CAD build for the part. Positions are in the model's coordinates, mm. A direction names the side the tool comes from. Coordinates: 2 decimals unless noted, no trailing zeros. Loops run counter-clockwise (first coordinate to the right, second up) from the corner with the lowest first, then second, coordinate; pieces in that order, holes last. Notation, with made-up numbers: (-37, -20.75) -> (-23, -20.75) arc R30 cw to (-23, 5.25) -> close; hole circle Ø9 at (52.25, 3.5). An arc over 180 degrees is marked (long way). Answer as a JSON object with one key per item and string values. Group by question number.
from build123d import *

# Parameters (mm, degrees)
SKETCH1_W           = 105.7
SKETCH1_H           = 105.7
SKETCH1_R           = 22.5
BOSS_EXTRUDE1_DEPTH = 10
SKETCH3_W           = 102
SKETCH3_H           = 102
SKETCH3_W_2         = 93
SKETCH3_H_2         = 93
CUT_EXTRUDE1_DEPTH  = 5
SKETCH8_R           = 3
CUT_EXTRUDE5_DEPTH  = 76.407194617
SKETCH4_R           = 10.375
CUT_EXTRUDE7_DEPTH  = 76.407194617
CUT_EXTRUDE11_DEPTH = 76.407194617
BOSS_EXTRUDE5_START = -40
SKETCH9_R           = 3
BOSS_EXTRUDE5_DEPTH = 40
CUT_EXTRUDE12_DEPTH = 47
CUT_EXTRUDE13_DEPTH = 2.5


with BuildPart() as part:
    # Sketch1 → Boss-Extrude1 (new body)
    with BuildSketch(Plane(origin=(0, 0, 0), x_dir=(1, 0, 0), z_dir=(0, 1, 0))):
        Rectangle(SKETCH1_W, SKETCH1_H)
        with Locations(Location((0, 0, 0), (0, 0, 270))):
            Circle(SKETCH1_R, mode=Mode.SUBTRACT)
    extrude(amount=BOSS_EXTRUDE1_DEPTH)

    # Sketch3 → Cut-Extrude1 (cut)
    with BuildSketch(Plane(origin=(0, 10, 0), x_dir=(1, 0, 0), z_dir=(0, 1, 0))):
        Rectangle(SKETCH3_W, SKETCH3_H)
        Rectangle(SKETCH3_W_2, SKETCH3_H_2, mode=Mode.SUBTRACT)
    extrude(amount=-CUT_EXTRUDE1_DEPTH, mode=Mode.SUBTRACT)

    # Sketch8 → Cut-Extrude5 (cut, through all)
    with BuildSketch(Plane.XZ.offset(-10)):
        with Locations(Location((-31.819805153, 31.819805153, 0), (0, 0, 270))):
            Circle(SKETCH8_R)
    extrude(amount=CUT_EXTRUDE5_DEPTH, mode=Mode.SUBTRACT)

    # Sketch4 → Cut-Extrude7 (cut, through all)
    with BuildSketch(Plane(origin=(0, 10, 0), x_dir=(1, 0, 0), z_dir=(0, 1, 0))):
        with Locations(Location((28.284271247, 28.284271247, 0), (0, 0, 270))):
            Circle(SKETCH4_R)
    extrude(amount=-CUT_EXTRUDE7_DEPTH, mode=Mode.SUBTRACT)

    # Sketch12 → Cut-Extrude11 (cut, through all)
    with BuildSketch(Plane.XZ):
        Polygon((43.899242251, -32.468290118), (39.71522338, -16.853319114), (24.100252377, -12.669300244), (12.669300244, -24.100252377), (16.853319114, -39.71522338), (32.468290118, -43.899242251), align=None)
    extrude(amount=-CUT_EXTRUDE11_DEPTH, mode=Mode.SUBTRACT)

    # Sketch9 → Boss-Extrude5 (add)
    with BuildSketch(Plane.XZ.offset(-10).offset(BOSS_EXTRUDE5_START)):
        Polygon((-23.44822625, 31.819805153), (-27.634015702, 39.069805153), (-36.005594605, 39.069805153), (-40.191384057, 31.819805153), (-36.005594605, 24.569805153), (-27.634015702, 24.569805153), align=None)
        with Locations(Location((-31.819805153, 31.819805153, 0), (0, 0, 270))):
            Circle(SKETCH9_R, mode=Mode.SUBTRACT)
    extrude(amount=BOSS_EXTRUDE5_DEPTH)

    # Sketch16 → Cut-Extrude12 (cut)
    with BuildSketch(Plane.XZ):
        Polygon((-25.757627327, 31.819805153), (-28.78871624, 37.069805153), (-34.850894067, 37.069805153), (-37.88198298, 31.819805153), (-34.850894067, 26.569805153), (-28.78871624, 26.569805153), align=None)
    extrude(amount=-CUT_EXTRUDE12_DEPTH, mode=Mode.SUBTRACT)

    # Sketch17 → Cut-Extrude13 (cut)
    with BuildSketch(Plane.XZ):
        Polygon((29.251441857, -14.049557305), (30.092603753, -10.91029837), (35.405195798, -12.333803118), (34.564033901, -15.473062053), align=None)
        Polygon((36.239222536, -40.128309832), (40.128309832, -36.239222536), (42.426406871, -38.537319575), (38.537319575, -42.426406871), align=None)
        Polygon((14.049557305, -29.251441857), (15.473062053, -34.564033901), (12.333803118, -35.405195798), (10.91029837, -30.092603753), align=None)
    extrude(amount=-CUT_EXTRUDE13_DEPTH, mode=Mode.SUBTRACT)


solid = part.part
Item 1: Band-saw the part on D-D, the plane x = -43. List the corners of the cut face in (y, z), and give its area (3 significant figures).
Item 2: Flat gauge pins, fed straight in: P1, Ø9, axis at x = -31.5, y = 31.5, coming from the -Z side; P2, Ø1.5, axis at x = -8.5, z = 38.5, coming from the +Y side; P3, Ø6.5, axis at x = -31, y = 27, coming from the +Z side. Where does each tip first touch, or does it go through?
Item 3: Band-saw the part on C-C, the plane y = 15.5. List the corners of the cut face in (x, z), and give its area (3 significant figures).
Item 4: Drill centre lines: L1, parallel to X at y = 6, z = 48.5; L2, parallel to X at y = 4, z = 0; L3, parallel to X at y = 9, z = -12.5. Where is each one in solid material? Low to high.
Item 5: Pull direction X, two halves, no side cores. Call faces 1 (the flat face through (52.85, 5, 1)), 2 (the flat face through (-21, 10, 10)), 3 (the flat face through (-51, 8, 1)): +X half, -X half, draft (parallel to the pull), parting line (faces both ways), or undercut.
Item 6: 3-axis set-ups, long thin cutter, end or side, ignore diameter. For faces 4 (the flat face through (-32, 30, 24.57)), 5 (the flat face through (-28, 50, 32)), 6 (the flat face through (12.458, 1.232, -29.678)), 7 (the flat face through (-1, 8, 51)): which of +Z, -Z, +X, -X, +Y, -Y reach the whole face in a straight line?
Item 7: Band-saw the part on A-A, the plane z = 0. List the corners of the cut face in (x, y), and give its area (3 significant figures).
Item 8: Band-saw the part on B-B, the plane x = 0. List the corners of the cut face in (y, z), and give its area (3 significant figures).
Reply:
{
 "1": {"outline": "(0, -52.85) -> (10, -52.85) -> (10, -51) -> (5, -51) -> (5, -46.5) -> (10, -46.5) -> (10, 46.5) -> (5, 46.5) -> (5, 51) -> (10, 51) -> (10, 52.85) -> (0, 52.85) -> close", "area": "1,010 mm²"},
 "2": {"P1": "z = 24.57", "P2": "y = 10", "P3": "z = 39.07"},
 "3": {"outline": "(-40.19, 31.82) -> (-36.01, 24.57) -> (-27.63, 24.57) -> (-23.45, 31.82) -> (-27.63, 39.07) -> (-36.01, 39.07) -> close; hole (-37.88, 31.82) -> (-34.85, 26.57) -> (-28.79, 26.57) -> (-25.76, 31.82) -> (-28.79, 37.07) -> (-34.85, 37.07) -> close", "area": "86.6 mm²"},
 "4": {"L1": "-52.85 to -51, 51 to 52.85", "L2": "-52.85 to -22.5, 22.5 to 52.85", "L3": "-52.85 to -51, -46.5 to -18.71, 18.71 to 46.5, 51 to 52.85"},
 "5": {"face 1": "+X half", "face 2": "draft", "face 3": "undercut"},
 "6": {"face 4": "-Z, +X, -X, +Y", "face 5": "+Z, -Z, +X, -X, +Y", "face 6": "-Y", "face 7": "+Y"},
 "7": {"outline": "(-52.85, 0) -> (-22.5, 0) -> (-22.5, 10) -> (-46.5, 10) -> (-46.5, 5) -> (-51, 5) -> (-51, 10) -> (-52.85, 10) -> close; (22.5, 0) -> (52.85, 0) -> (52.85, 10) -> (51, 10) -> (51, 5) -> (46.5, 5) -> (46.5, 10) -> (22.5, 10) -> close", "area": "562 mm²"},
 "8": {"outline": "(0, -52.85) -> (10, -52.85) -> (10, -51) -> (5, -51) -> (5, -46.5) -> (10, -46.5) -> (10, -22.5) -> (0, -22.5) -> close; (0, 22.5) -> (10, 22.5) -> (10, 46.5) -> (5, 46.5) -> (5, 51) -> (10, 51) -> (10, 52.85) -> (0, 52.85) -> close", "area": "562 mm²"}
}
